from build123d import *

# Parameters (mm, degrees)
SALIENTE_EXTRUIR1_DEPTH    = 40
CROQUIS2_R                 = 1.6
CORTAR_EXTRUIR1_DEPTH      = 6
CORTAR_EXTRUIR2_DEPTH      = 3
CORTAR_EXTRUIR3_DEPTH      = 6
REDONDEO1_R                = 4
REDONDEO2_R                = 2
REDONDEO3_R                = 1
CROQUIS5_R                 = 12.5
CORTAR_EXTRUIR4_DEPTH      = 8.5
CORTAR_EXTRUIR4_DEPTH_BACK = 8.5


with BuildPart() as part:
    # Croquis1 → Saliente-Extruir1 (new body)
    with BuildSketch(Plane(origin=(0, 0, 0), x_dir=(1, 0, 0), z_dir=(0, 1, 0))):
        with BuildLine():
            Line((-17.5, -7.5), (7.5, -7.5))
            Line((7.5, -7.5), (7.5, -3.6))
            Line((7.5, -3.6), (0, -3.6))
            ThreePointArc((0, -3.6), (-3.6, 0), (0, 3.6))
            Line((0, 3.6), (6.57951366, 3.6))
            ThreePointArc((6.57951366, 3.6), (-1.857908441, 7.266235354), (-7.5, 0))
            Line((-7.5, 0), (-7.5, -2.5))
            Line((-7.5, -2.5), (-17.5, -2.5))
            Line((-17.5, -2.5), (-17.5, -7.5))
        make_face()
    extrude(amount=SALIENTE_EXTRUIR1_DEPTH)

    # Croquis2 → Cortar-Extruir1 (cut, through all)
    with BuildSketch(Plane(origin=(0, 0, 2.5), x_dir=(-1, 0, 0), z_dir=(0, 0, -1))):
        with Locations((12.5, 7)):
            Circle(CROQUIS2_R)
        with Locations((12.5, 33)):
            Circle(CROQUIS2_R)
    extrude(amount=-CORTAR_EXTRUIR1_DEPTH, mode=Mode.SUBTRACT)

    # Croquis3 → Cortar-Extruir2 (cut)
    with BuildSketch(Plane(origin=(0, 0, 2.5), x_dir=(-1, 0, 0), z_dir=(0, 0, -1))):
        Polygon((15.3, 31.383419246), (15.3, 34.616580754), (12.5, 36.233161507), (9.7, 34.616580754), (9.7, 31.383419246), (12.5, 29.766838493), align=None)
        Polygon((12.5, 10.233161507), (15.3, 8.616580754), (15.3, 5.383419246), (12.5, 3.766838493), (9.7, 5.383419246), (9.7, 8.616580754), align=None)
    extrude(amount=-CORTAR_EXTRUIR2_DEPTH, mode=Mode.SUBTRACT)

    # Croquis4 → Cortar-Extruir3 (cut, through all)
    with BuildSketch(Plane(origin=(0, 0, 2.5), x_dir=(-1, 0, 0), z_dir=(0, 0, -1))):
        with BuildLine():
            Line((17.5, 27.5), (17.5, 12.5))
            ThreePointArc((17.5, 12.5), (10, 20), (17.5, 27.5))
        make_face()
    extrude(amount=-CORTAR_EXTRUIR3_DEPTH, mode=Mode.SUBTRACT)

    # Redondeo1
    redondeo1_edges = [part.edges().sort_by_distance(p)[0] for p in [
        (-17.5, 40, 5),
        (-17.5, 12.5, 5),
        (-17.5, 27.5, 5),
        (-17.5, 0, 5),
    ]]
    fillet(redondeo1_edges, radius=REDONDEO1_R)

    # Redondeo2
    redondeo2_edges = [part.edges().sort_by_distance(p)[0] for p in [
        (7.5, 20, 7.5),
        (-7.5, 20, 2.5),
    ]]
    fillet(redondeo2_edges, radius=REDONDEO2_R)

    # Redondeo3
    redondeo3_edges = [part.edges().sort_by_distance(p)[0] for p in [
        (7.5, 20, 3.6),
        (6.57951366, 20, -3.6),
    ]]
    fillet(redondeo3_edges, radius=REDONDEO3_R)

    # Croquis5 → Cortar-Extruir4 (cut, two sides)
    with BuildSketch(Plane.XY) as cortar_extruir4_sk:
        with Locations((10, 20)):
            Circle(CROQUIS5_R)
    extrude(amount=CORTAR_EXTRUIR4_DEPTH, mode=Mode.SUBTRACT)
    extrude(cortar_extruir4_sk.sketch, amount=-CORTAR_EXTRUIR4_DEPTH_BACK, mode=Mode.SUBTRACT)


solid = part.part
Verification items for the finished model (mm, model axes). A direction names the side the tool comes from. Coordinates: 2 decimals unless noted, no trailing zeros. Write each loop counter-clockwise with the first axis right and the second up, starting at its lowest first coordinate (ties: lowest second). Pieces come first, ordered by that corner, then holes. Notation, with made-up numbers: M 2.5,-34.5 L 32.5,-34.5 A20 ccw 32.5,-26.5 Z; hole C 70,67.25 d5. An arc over 180 degrees is marked long. Use CSV: the item, a comma, the result in double quotes.
Q1. Thickness scan on line 1 along Y through (x, z) = (-12.5, 6.15); line 2 along Z through (x, y) = (-12.75, 11); line 3 along X through (y, z) = (17.5, 0.25). Record the ranges inside material, lowest first. Write a range as [from, to].
Computed values:
line 1,"[0, 5.4], [8.6, 14.41], [25.59, 31.4], [34.6, 40]"
line 2,"[2.5, 7.5]"
line 3,"[-7.5, -3.59]"
Q2. Set-up check for faces 5 (the flat face through (3, 35, 3.6)), 6 (the flat face through (-11.08, 30.586, 3.979)), 7 (the cylindrical face through (-16.803, 28.526, 5.035)): record each of +Z, -Z, +X, -X, +Y, -Y from which the full face is reachable in a straight line by a thin tool's end or side.
Computed values:
face 5,"+X, +Y, -Y"
face 6,"-Z"
face 7,"+Z, -Z, -X"
Q3. Section check B-B, the plane y = 7. Enter the section's corners in (x, z).
Computed values:
outline,"M -17.5,2.5 L -15.3,2.5 L -15.3,5.5 L -14.1,5.5 L -14.1,7.5 L -17.5,7.5 Z; M -10.9,5.5 L -9.7,5.5 L -9.7,2.5 L -9.5,2.5 A2 cw -7.5,0.5 L -7.5,0 A7.5 ccw 5.3,-5.31 A1 ccw 4.59,-3.6 L 0,-3.6 A3.6 cw 0,3.6 L 6.5,3.6 A1 ccw 7.5,4.6 L 7.5,5.5 A2 ccw 5.5,7.5 L -10.9,7.5 Z"
Q4. Go/stop test with flat-tipped pins: P1, Ø5, axis at x = 4.5, y = 8, coming from the -Z side; P2, Ø4.5, axis at x = -12.5, y = 32, coming from the -Z side; P3, Ø1.7, axis at x = -13.5, y = 8, coming from the -Z side. Record where each tip stops, or that it passes through.
Computed values:
P1,"z = -7.23"
P2,"z = 2.5"
P3,"z = 5.5"
Q5. Section check A-A, the plane z = 5. Enter the section's corners in (x, y), and give its area (3 significant figures).
Computed values:
outline,"M -17.5,4 A4 ccw -13.5,0 L 7.5,0 L 7.5,7.75 A12.5 cw 7.5,32.25 L 7.5,40 L -13.5,40 A4 ccw -17.5,36 L -17.5,30.78 A4 ccw -14.89,27.03 A7.5 cw -14.89,12.97 A4 ccw -17.5,9.22 Z; hole M -15.3,5.38 L -12.5,3.77 L -9.7,5.38 L -9.7,8.62 L -12.5,10.23 L -15.3,8.62 Z; hole M -15.3,31.38 L -12.5,29.77 L -9.7,31.38 L -9.7,34.62 L -12.5,36.23 L -15.3,34.62 Z"
area,"663 mm²"
Q6. Mould release check, pull along Y, two halves, no side actions. Record for faces 1 (the cylindrical face through (-2.5, 20.2, -5)), 2 (the flat face through (-6, 20, 7.5)), 3 (the flat face through (-3, 0, 3)), 4 (the cylindrical face through (-16.764, 11.53, 5.035)): pulls with the +Y half, pulls with the -Y half, needs draft (parallel to the pull), parting line crosses it, or undercut.
Computed values:
face 1,"undercut"
face 2,"needs draft"
face 3,"pulls with the -Y half"
face 4,"undercut"
Q7. Section check D-D, the plane y = 28. Enter the section's corners in (x, z).
Computed values:
outline,"M -16.37,2.5 L -9.5,2.5 A2 cw -7.5,0.5 L -7.5,0 A7.5 ccw 0.4,-7.49 L 0.4,-3.6 L 0,-3.6 A3.6 cw 0,3.6 L 0.4,3.6 L 0.4,7.5 L -16.37,7.5 Z"
Q8. Section check C-C, the plane x = 3.75. Enter the section's corners in (y, z).
Computed values:
outline,"M 0,-6.5 L 9.17,-6.5 L 9.17,-3.6 L 0,-3.6 Z; M 0,3.6 L 9.17,3.6 L 9.17,7.5 L 0,7.5 Z; M 30.83,-6.5 L 40,-6.5 L 40,-3.6 L 30.83,-3.6 Z; M 30.83,3.6 L 40,3.6 L 40,7.5 L 30.83,7.5 Z"
